from build123d import *

# Parameters (mm, degrees)
SKETCH1_R           = 27.5
BOSS_EXTRUDE1_DEPTH = 7
SKETCH4_R           = 20.05
CUT_EXTRUDE1_DEPTH  = 5
SKETCH5_R           = 18.05
CUT_EXTRUDE2_DEPTH  = 40.210967853
BOSS_EXTRUDE2_START = 24
SKETCH6_R           = 30
SKETCH6_R_2         = 20.05
BOSS_EXTRUDE2_DEPTH = 24
SKETCH7_R           = 25.05
CUT_EXTRUDE3_DEPTH  = 22
SKETCH8_R           = 22.75
CUT_EXTRUDE4_DEPTH  = 5
SKETCH9_R           = 25.8445
CUT_EXTRUDE5_DEPTH  = 8
SKETCH10_OUTSIDE_W  = 80.068
SKETCH10_OUTSIDE_H  = 80.068
SKETCH10_OUTSIDE_R  = 25.8445
CUT_EXTRUDE6_DEPTH  = 3
CHAMFER3_SIZE       = 2
CHAMFER4_SIZE       = 1
CHAMFER5_SIZE       = 1


with BuildPart() as part:
    # Sketch1 → Boss-Extrude1 (new body)
    with BuildSketch(Plane.XY):
        Circle(SKETCH1_R)
    extrude(amount=BOSS_EXTRUDE1_DEPTH)

    # Sketch4 → Cut-Extrude1 (cut)
    with BuildSketch(Plane.XY.offset(7)):
        Circle(SKETCH4_R)
    extrude(amount=-CUT_EXTRUDE1_DEPTH, mode=Mode.SUBTRACT)

    # Sketch5 → Cut-Extrude2 (cut, through all)
    with BuildSketch(Plane.XY.offset(2)):
        Circle(SKETCH5_R)
    extrude(amount=-CUT_EXTRUDE2_DEPTH, mode=Mode.SUBTRACT)

    # Sketch6 → Boss-Extrude2 (add)
    with BuildSketch(Plane.XY.offset(7).offset(BOSS_EXTRUDE2_START)):
        Circle(SKETCH6_R)
        Circle(SKETCH6_R_2, mode=Mode.SUBTRACT)
    extrude(amount=-BOSS_EXTRUDE2_DEPTH)

    # Sketch7 → Cut-Extrude3 (cut)
    with BuildSketch(Plane.XY.offset(31)):
        Circle(SKETCH7_R)
    extrude(amount=-CUT_EXTRUDE3_DEPTH, mode=Mode.SUBTRACT)

    # Sketch8 → Cut-Extrude4 (cut)
    with BuildSketch(Plane.XY.offset(9)):
        Circle(SKETCH8_R)
    extrude(amount=-CUT_EXTRUDE4_DEPTH, mode=Mode.SUBTRACT)

    # Sketch9 → Cut-Extrude5 (cut)
    with BuildSketch(Plane.XY.offset(31)):
        Circle(SKETCH9_R)
    extrude(amount=-CUT_EXTRUDE5_DEPTH, mode=Mode.SUBTRACT)

    # Sketch10 outside → Cut-Extrude6 (cut)
    with BuildSketch(Plane(origin=(0, 0, 0), x_dir=(-1, 0, 0), z_dir=(0, 0, -1))):
        Rectangle(SKETCH10_OUTSIDE_W, SKETCH10_OUTSIDE_H)
        with Locations(Location((0, 0, 0), (0, 0, 180))):
            Circle(SKETCH10_OUTSIDE_R, mode=Mode.SUBTRACT)
    extrude(amount=-CUT_EXTRUDE6_DEPTH, mode=Mode.SUBTRACT)

    # Chamfer3
    chamfer3_edges = [part.edges().sort_by_distance(p)[0] for p in [
        (-30, 0, 7),
    ]]
    chamfer(chamfer3_edges, length=CHAMFER3_SIZE)

    # Chamfer4
    chamfer4_edges = [part.edges().sort_by_distance(p)[0] for p in [
        (-27.5, 0, 3),
    ]]
    chamfer(chamfer4_edges, length=CHAMFER4_SIZE)

    # Chamfer5
    chamfer5_edges = [part.edges().sort_by_distance(p)[0] for p in [
        (-18.05, 0, 0),
        (-30, 0, 31),
        (-25.8445, 0, 31),
    ]]
    chamfer(chamfer5_edges, length=CHAMFER5_SIZE)


solid = part.part
Geometry check sheet. Reference: the model listing, model coordinates, mm. A direction names the side the tool comes from. Give positions to 0.01 mm unless a question says otherwise; leave off trailing zeros. Loops run counter-clockwise (first coordinate to the right, second up) from the corner with the lowest first, then second, coordinate; pieces in that order, holes last.
(1) Depth check by flat-ended pin: pin 1 Ø17 at (x, y) = (-11, -10.5) entering from -Z; pin 2 Ø10 at (x, y) = (-5, 20.5) entering from +Z; pin 3 Ø6 at (y, z) = (13, 14.5) entering from +X; pin 4 Ø1.5 at (x, z) = (24, 28) entering from +Y. Enter the tip coordinate at first touch or a pass-through.
From the geometry:
pin 1: stops at z = 0
pin 2: stops at z = 30.26
pin 3: stops at x = 28.28
pin 4: stops at y = 18.96
(2) Set-up check for faces 1 (the flat face through (11, -20.3, 9)), 2 (the flat face through (-12, -15, 0)), 3 (the flat face through (18.5, -20.6, 7)): record each of +Z, -Z, +X, -X, +Y, -Y from which the full face is reachable in a straight line by a thin tool's end or side.
From the geometry:
face 1: +Z
face 2: -Z, +X, -X, +Y, -Y
face 3: -Z
(3) Section check A-A on z = 19. Record the cut outline in (x, y), then the cut area to 3 significant figures.
From the geometry:
outline: circle Ø60 at (0, 0); hole circle Ø50.1 at (0, 0)
area: 856 mm2
(4) Thickness scan on L1, parallel to Y at x = 0, z = 26; L2, parallel to Z at x = -18.5, y = -17; L3, parallel to Z at x = 18.5, y = -8. Record the ranges inside material, lowest first.
From the geometry:
L1: y = -30 to -25.84, 25.84 to 30
L2: z = 0 to 23
L3: z = 0 to 4
(5) Release check for a two-part mould opening along Y. For faces 4 (the cylindrical face through (-5.961, -26.846, 5.479)), 5 (the flat face through (-5.8, -25.4, 3)), 6 (the cylindrical face through (-15.91, -12.2, 3.01)) record: released by +Y, released by -Y, zero draft, split by the parting line, or undercut.
From the geometry:
face 4: split by the parting line
face 5: zero draft
face 6: undercut
